Autodesk Fusion 360 part; units mm, degrees
sketch "Boceto1" plane through (0, 0, 0) normal (1, 0, 0) x (0, 1, 0)
  line L0 (0, 0) -> (0, 15)
  line L1 (0, 0) -> (-15, 0)
  arc A0 (-15, 0) -> (0, 15) centre (-26.7073, 26.7073) ccw
  dimension "d1" = 15
  dimension "d2" = 15
extrude "Extruir1" add sketch "Boceto1" along normal blind 50
sketch "Boceto2" plane through (0, 0, 0) normal (0, 1, 0) x (-1, 0, 0)
  line L0 (0, 0) -> (0, 15)
  line L1 (0, 15) -> (-50, 15)
  line L2 (-50, 15) -> (-50, 0)
  line L3 (-50, 0) -> (0, 0)
  circle A0 centre (-33.75, 10.6) radius 1.75
  circle A1 centre (-16.25, 10.6) radius 1.75
  dimension "d9" = 3.5
  dimension "d14" = 3.5
extrude "Extruir2" cut sketch "Boceto2" against normal blind 5 contours A0 | A1
sketch "Boceto3" plane through (0, 0, 0) normal (0, 0, -1) x (1, 0, 0)
  line L0 (0, 15) -> (0, 0)
  line L1 (0, 0) -> (50, 0)
  line L2 (50, 0) -> (50, 15)
  line L3 (50, 15) -> (0, 15)
  circle A0 centre (10, 5) radius 1.6
  circle A1 centre (40, 5) radius 1.6
  dimension "d19" = 3.2
  dimension "d22" = 3.2
extrude "Extruir3" cut sketch "Boceto3" against normal blind 11 contours A0 | A1
Model file for the job. Use its own axes, mm. Coordinates: 2 decimals unless noted, no trailing zeros. Order: outer loops, then holes, each group sorted by start corner. A loop starts at its lowest first (then second) coordinate and runs counter-clockwise, first axis right, second up. Notation, with made-up numbers: (24, -12) -> (42, -12) arc R25 cw to (42, 11) -> close; hole circle Ø6 at (78, 63.25). An arc over 180 degrees is marked (long way). Answer as a JSON object with one key per item and string values. Group by question number.
1) Pull direction Z, two halves, no side cores. Call faces 1 (the face through (16.63, -1.4, 8.89)), 2 (the face through (24.65, -5.98, 6.195)), 3 (the face through (50, -4, 4)): +Z half, -Z half, draft (parallel to the pull), parting line (faces both ways), or undercut.
2) Cut at C-C, the plane z = 10.6. Write the cut outline in (x, y).
3) Cut at D-D, the plane z = 3.75. Write the cut outline in (x, y).
4) Cut at B-B, the plane x = 33.75. Write the cut outline in (y, z), then the cut area to 3 significant figures.
5) Drill centre lines: L1, parallel to X at y = -5, z = 6.25; L2, parallel to X at y = -0.8, z = 10.6; L3, parallel to Z at x = 33.75, y = -1.9. Where is each one in solid material? Low to high.
6) Flat gauge pins, fed straight in: pin 1 (1.5 mm diameter, centred on x = 35, z = 11.5, fed in from -Y); pin 2 (2 mm diameter, centred on x = 33.75, z = 10.6, fed in from -Y); pin 3 (5 mm diameter, centred on x = 40, y = -5, fed in from +Z); pin 4 (8 mm diameter, centred on x = 13.5, y = -7, fed in from +Z). Where does each tip first touch, or does it go through?
7) Cut at A-A, the plane y = -5. Write the cut outline in (x, z), then the cut area to 3 significant figures.
Check values:
{
 "1": {"face 1": "undercut", "face 2": "+Z half", "face 3": "draft"},
 "2": {"outline": "(0, -2.4) -> (14.5, -2.4) -> (14.5, 0) -> (0, 0) -> close; (18, -2.4) -> (32, -2.4) -> (32, 0) -> (18, 0) -> close; (35.5, -2.4) -> (50, -2.4) -> (50, 0) -> (35.5, 0) -> close"},
 "3": {"outline": "(0, -8.73) -> (50, -8.73) -> (50, 0) -> (0, 0) -> close; hole circle Ø3.2 at (10, -5); hole circle Ø3.2 at (40, -5)"},
 "4": {"outline": "(-15, 0) -> (0, 0) -> (0, 8.85) -> (-3.65, 8.85) arc R29.16 cw to start; (-1.33, 12.35) -> (0, 12.35) -> (0, 15) arc R29.16 cw to start", "area": "75.6 mm²"},
 "5": {"L1": "x = 0 to 8.4, 11.6 to 38.4, 41.6 to 50", "L2": "x = 0 to 14.5, 18 to 32, 35.5 to 50", "L3": "z = 0 to 8.85"},
 "6": {"pin 1": "stops at y = -2.19", "pin 2": "passes through", "pin 3": "stops at z = 10.45", "pin 4": "stops at z = 9.73"},
 "7": {"outline": "(0, 0) -> (8.4, 0) -> (8.4, 7.24) -> (0, 7.24) -> close; (11.6, 0) -> (38.4, 0) -> (38.4, 7.24) -> (11.6, 7.24) -> close; (41.6, 0) -> (50, 0) -> (50, 7.24) -> (41.6, 7.24) -> close", "area": "315 mm²"}
}
